```python
from build123d import *

# Parameters (mm, degrees)
BOSS_EXTRUDE1_DEPTH = 457.2
CUT_EXTRUDE1_DEPTH  = 914.4


with BuildPart() as part:
    # Sketch1 → Boss-Extrude1 (new body, symmetric)
    with BuildSketch(Plane.XY):
        with BuildLine():
            Line((19.05, 31.75), (-19.05, 31.75))
            ThreePointArc((-19.05, 31.75), (-28.030256121, 28.030256121), (-31.75, 19.05))
            Line((-31.75, 19.05), (-31.75, -19.05))
            ThreePointArc((-31.75, -19.05), (-28.030256121, -28.030256121), (-19.05, -31.75))
            Line((-19.05, -31.75), (19.05, -31.75))
            ThreePointArc((19.05, -31.75), (28.030256121, -28.030256121), (31.75, -19.05))
            Line((31.75, -19.05), (31.75, 19.05))
            ThreePointArc((31.75, 19.05), (28.030256121, 28.030256121), (19.05, 31.75))
        make_face()
        with BuildLine():
            ThreePointArc((-25.4, -19.05), (-23.540128061, -23.540128061), (-19.05, -25.4))
            Line((-19.05, -25.4), (19.05, -25.4))
            ThreePointArc((19.05, -25.4), (23.540128061, -23.540128061), (25.4, -19.05))
            Line((25.4, -19.05), (25.4, 19.05))
            ThreePointArc((25.4, 19.05), (23.540128061, 23.540128061), (19.05, 25.4))
            Line((19.05, 25.4), (-19.05, 25.4))
            ThreePointArc((-19.05, 25.4), (-23.540128061, 23.540128061), (-25.4, 19.05))
            Line((-25.4, 19.05), (-25.4, -19.05))
        make_face(mode=Mode.SUBTRACT)
    extrude(amount=BOSS_EXTRUDE1_DEPTH, both=True)

    # Sketch2 → Cut-Extrude1 (cut)
    with BuildSketch(Plane(origin=(31.75, 0, 0), x_dir=(0, 0, -1), z_dir=(1, 0, 0))):
        Polygon((457.2, 31.75), (457.2, -68.178184421), (444.044204942, -68.178184421), align=None)
    extrude(amount=-CUT_EXTRUDE1_DEPTH, mode=Mode.SUBTRACT)


solid = part.part
```
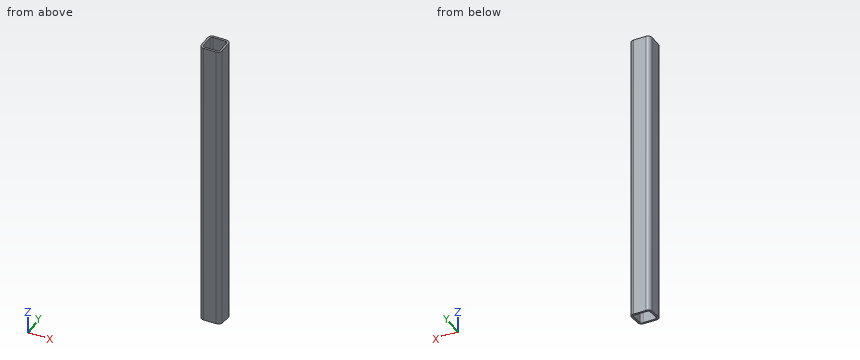
The listing builds one solid part. Answer for the finished solid, in the listing's coordinates (mm). Round coordinates to 2 decimals unless told otherwise and drop trailing zeros. Loops run counter-clockwise (first coordinate to the right, second up) from the corner with the lowest first, then second, coordinate; pieces in that order, holes last.
Q1. Section B-B, the plane z = -205 is taken. Determine the outline of the cut face in (x, y), then the cut area to 3 significant figures.
Q2. Find the intervals of material crossed by line 1 (X direction, y = -8, z = 104.5); line 2 (Y direction, x = -19.5, z = 216.5), in increasing order.
Q3. Given pin 1 Ø8 at (y, z) = (25, -134) entering from -X; pin 2 Ø5 at (y, z) = (-21, -4.5) entering from -X; pin 3 Ø1 at (y, z) = (23.5, 97) entering from -X, each flat-ended and moving along its own axis, determine where each tip first touches the part or whether it passes through.
Q4. Section A-A, the plane x = -2.5 is taken. Determine the outline of the cut face in (y, z), then the cut area to 3 significant figures.
Q5. Section C-C, the plane y = -10 is taken. Determine the outline of the cut face in (x, z), then the cut area to 3 significant figures.
Completed:
1. outline: (-31.75, -19.05) arc R12.7 ccw to (-19.05, -31.75) - (19.05, -31.75) arc R12.7 ccw to (31.75, -19.05) - (31.75, 19.05) arc R12.7 ccw to (19.05, 31.75) - (-19.05, 31.75) arc R12.7 ccw to (-31.75, 19.05) - close; hole (-25.4, -19.05) arc R6.35 ccw to (-19.05, -25.4) - (19.05, -25.4) arc R6.35 ccw to (25.4, -19.05) - (25.4, 19.05) arc R6.35 ccw to (19.05, 25.4) - (-19.05, 25.4) arc R6.35 ccw to (-25.4, 19.05) - close
1. area: 1,350 mm2
2. line 1: x = -31.75 to -25.4, 25.4 to 31.75
2. line 2: y = -31.74 to -25.38, 25.38 to 31.74
3. pin 1: stops at x = -31.6
3. pin 2: stops at x = -31.75
3. pin 3: stops at x = -31.12
4. outline: (-31.75, -448.84) - (-25.4, -449.68) - (-25.4, 457.2) - (-31.75, 457.2) - close; (25.4, -456.36) - (31.75, -457.2) - (31.75, 457.2) - (25.4, 457.2) - close
4. area: 11,600 mm2
5. outline: (-31.75, -451.7) - (-25.4, -451.7) - (-25.4, 457.2) - (-31.75, 457.2) - close; (25.4, -451.7) - (31.75, -451.7) - (31.75, 457.2) - (25.4, 457.2) - close
5. area: 11,500 mm2
